Geometry check sheet. Reference: drawing and pictorial views, mm from the part's lowest x, y, z. Give positions to 0.01 mm unless a question says otherwise; leave off trailing zeros. Write each loop counter-clockwise with the first axis right and the second up, starting at its lowest first coordinate (ties: lowest second). Pieces come first, ordered by that corner, then holes. Notation, with made-up numbers: (23.25, -36.5) -> (37.25, -36.5) arc R18 ccw to (37.25, -30.5) -> close; hole circle Ø5 at (32.5, 2). An arc over 180 degrees is marked (long way). Return JSON: item names as keys, results as strings.
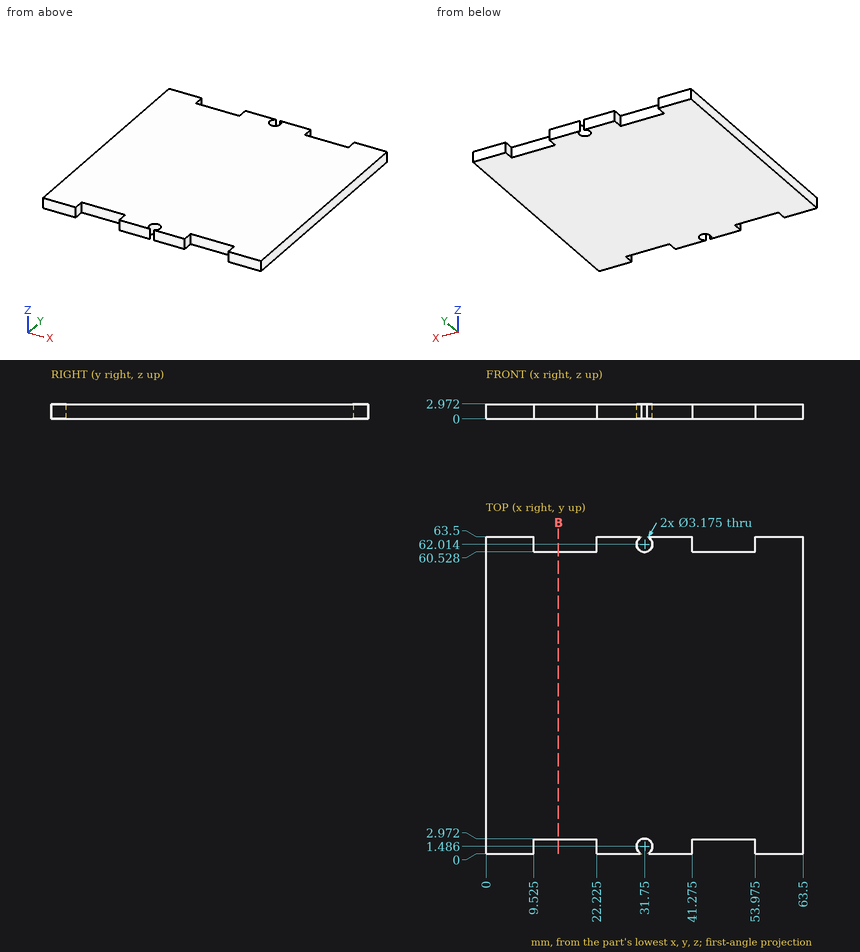
(1) Cross-section at B-B on x = 14.5. Enter the section's corners in (y, z), then the cut area to 3 significant figures.
Reply:
{"outline": "(2.97, 0) -> (60.53, 0) -> (60.53, 2.97) -> (2.97, 2.97) -> close", "area": "171 mm^2"}
(2) Thickness scan on L1, parallel to Y at x = 50, z = 0.4; L2, parallel to Y at x = 31.75, z = 1.15. Record the ranges inside material, lowest first.
Reply:
{"L1": "2.97 to 60.53", "L2": "3.07 to 60.43"}
(3) Depth check by flat-ended pin: pin 1 Ø1.5 at (x, z) = (15, 1) entering from +Y. Enter the tip coordinate at first touch or a pass-through.
Reply:
{"pin 1": "y = 60.53"}
